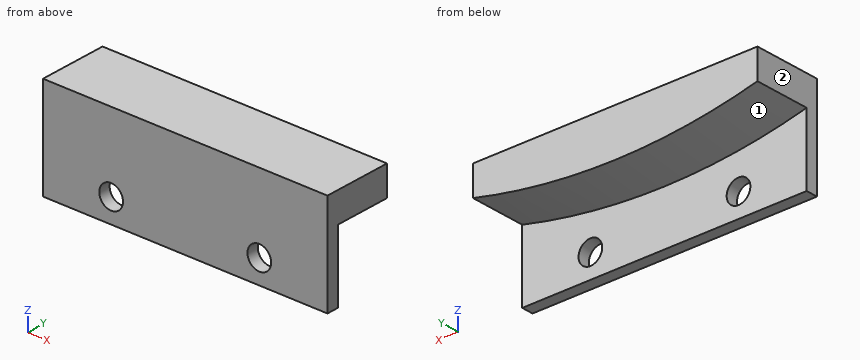
from build123d import *

# Parameters (mm, degrees)
BOSS_EXTRUDE1_DEPTH = 11.525
SKETCH1_3_R         = 2
BOSS_EXTRUDE2_DEPTH = 2


with BuildPart() as part:
    # Sketch1 → Boss-Extrude1 (new body)
    with BuildSketch(Plane(origin=(0, 0, 0), x_dir=(1, 0, 0), z_dir=(0, 1, 0))):
        with BuildLine():
            ThreePointArc((-24, 5), (0, 7.922711204), (24, 5))
            Line((24, 5), (24, 0))
            Line((24, 0), (-24, 0))
            Line((-24, 0), (-24, 5))
        make_face()
    extrude(amount=BOSS_EXTRUDE1_DEPTH)

    # Sketch1_3 → Boss-Extrude2 (add)
    # profile 1 of 2: a face of its own
    with BuildSketch(Plane(origin=(0, 0, 0), x_dir=(1, 0, 0), z_dir=(0, 1, 0))):
        with BuildLine():
            Line((-24, 5), (-24, 0))
            Line((-24, 0), (24, 0))
            Line((24, 0), (24, 5))
            ThreePointArc((24, 5), (0, 7.922711204), (-24, 5))
        make_face()
    # profile 2 of 2: a face of its own
    with BuildSketch(Plane(origin=(0, 0, 0), x_dir=(1, 0, 0), z_dir=(0, 1, 0))):
        with BuildLine():
            Line((-24, 17), (-24, 5))
            ThreePointArc((-24, 5), (0, 7.922711204), (24, 5))
            Line((24, 5), (24, 17))
            Line((24, 17), (-24, 17))
        make_face()
        with Locations(Location((-12.5, 13, 0), (0, 0, 270))):
            Circle(SKETCH1_3_R, mode=Mode.SUBTRACT)
        with Locations(Location((12.5, 13, 0), (0, 0, 270))):
            Circle(SKETCH1_3_R, mode=Mode.SUBTRACT)
    extrude(amount=BOSS_EXTRUDE2_DEPTH)


solid = part.part
Read the model definition and answer for the solid it produces. Units are mm, in the model's axes. Face numbers are marked on the shaded views. A direction names the side the tool comes from. Round coordinates to 2 decimals unless told otherwise and drop trailing zeros. Write each loop counter-clockwise with the first axis right and the second up, starting at its lowest first coordinate (ties: lowest second). Pieces come first, ordered by that corner, then holes. Notation, with made-up numbers: (14.5, 36) - (60.5, 36) arc R18 ccw to (60.5, 49) - close; hole circle Ø7 at (-31, -20). An arc over 180 degrees is marked (long way). Use a Markdown table: item, result.
(1) Straight lines are drawn through the part: line 1 along X through (y, z) = (1.1, -13); line 2 along Y through (x, z) = (-3, -14.5); line 3 along Z through (x, y) = (-14, 1). For each, find the intervals that lie inside material, in ascending order. Write a range as [from, to].
Reported:
| item | result |
|---|---|
| line 1 | [-24, -14.5], [-10.5, 10.5], [14.5, 24] |
| line 2 | [0, 2] |
| line 3 | [-17, -14.32], [-11.68, 0] |
(2) The part is cut by section B-B (x = 12.5). Write down the section's boundary in (y, z) (3 decimals).
Reported:
| item | result |
|---|---|
| outline | (0, -17) - (2, -17) - (2, -15) - (0, -15) - close; (0, -11) - (2, -11) - (2, -7.138) - (11.525, -7.138) - (11.525, 0) - (0, 0) - close |
(3) Each of these flat-tipped pins is pushed along its axis until it touches: pin 1 Ø4.5 at (x, z) = (12.5, -13) entering from +Y; pin 2 Ø3 at (x, y) = (0.5, 6) entering from -Z. Where does it stop, or does it pass through?
Reported:
| item | result |
|---|---|
| pin 1 | y = 2 |
| pin 2 | z = -7.92 |
(4) The part is cut by section A-A (z = -13). Write down the section's boundary in (x, y).
Reported:
| item | result |
|---|---|
| outline | (-24, 0) - (-14.5, 0) - (-14.5, 2) - (-24, 2) - close; (-10.5, 0) - (10.5, 0) - (10.5, 2) - (-10.5, 2) - close; (14.5, 0) - (24, 0) - (24, 2) - (14.5, 2) - close |
(5) The part is cut by section D-D (y = 6). Write down the section's boundary in (x, z).
Reported:
| item | result |
|---|---|
| outline | (-24, -5) arc R100 ccw to (24, -5) - (24, 0) - (-24, 0) - close |
(6) Which of the six approach directions +Z, -Z, +X, -X, +Y, -Y give full straight-line access (tool end or side, diameter ignored) to the marked faces 1 and 2?
Reported:
| item | result |
|---|---|
| face 1 | -Z, +Y |
| face 2 | +Z, -Z, -X, +Y, -Y |
